Source: CAD feature listing. Evaluate the final solid. Frame: model axes, mm. Coordinates: 2 decimals unless noted, no trailing zeros. Loops run counter-clockwise (first coordinate to the right, second up) from the corner with the lowest first, then second, coordinate; pieces in that order, holes last.
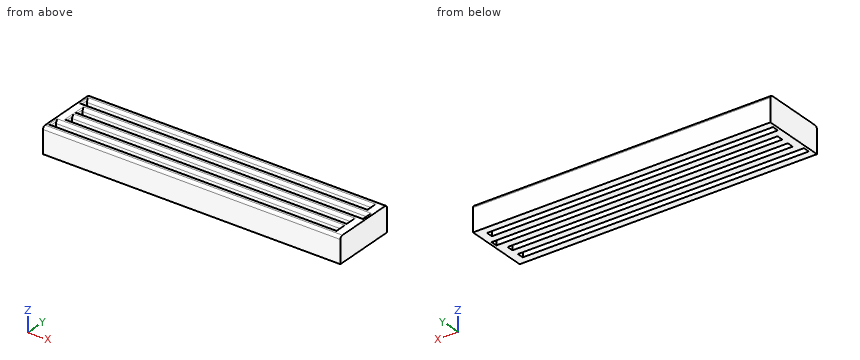
from build123d import *

# Parameters (mm, degrees)
SKETCH003_W   = 53.9
SKETCH003_H   = 11.48
SKETCH003_W_2 = 51.85
SKETCH003_H_2 = 1.194
SKETCH003_W_3 = 50.8
PAD001_DEPTH  = 4.67
FILLET_R      = 0.5
FILLET001_R   = 0.5
FILLET002_R   = 0.5
FILLET003_R   = 0.5
FILLET004_R   = 0.5
FILLET005_R   = 0.5
FILLET006_R   = 0.5
FILLET007_R   = 0.5
FILLET008_R   = 0.5
FILLET009_R   = 0.5
FILLET010_R   = 0.2
FILLET011_R   = 0.2
FILLET012_R   = 0.2
FILLET013_R   = 0.2
FILLET014_R   = 0.2
FILLET015_R   = 0.2
FILLET016_R   = 0.2
FILLET017_R   = 0.19


with BuildPart() as part:
    # Sketch003 → Pad001 (new body)
    with BuildSketch(Plane.XY.offset(0.28)):
        with Locations((27.89, 7.34)):
            Rectangle(SKETCH003_W, SKETCH003_H)
        with Locations((27.365, 11.1422)):
            Rectangle(SKETCH003_W_2, SKETCH003_H_2, mode=Mode.SUBTRACT)
        with Locations((28.415, 8.6074)):
            Rectangle(SKETCH003_W_2, SKETCH003_H_2, mode=Mode.SUBTRACT)
        with Locations((27.89, 6.0726)):
            Rectangle(SKETCH003_W_3, SKETCH003_H_2, mode=Mode.SUBTRACT)
        with Locations((27.365, 3.5378)):
            Rectangle(SKETCH003_W_2, SKETCH003_H_2, mode=Mode.SUBTRACT)
    extrude(amount=PAD001_DEPTH)

    # Fillet
    fillet_edges = [part.edges().sort_by_distance(p)[0] for p in [
        (27.89, 1.6, 4.95),
    ]]
    fillet(fillet_edges, radius=FILLET_R)

    # Fillet001
    fillet001_edges = [part.edges().sort_by_distance(p)[0] for p in [
        (27.365, 2.9408, 4.95),
    ]]
    fillet(fillet001_edges, radius=FILLET001_R)

    # Fillet002
    fillet002_edges = [part.edges().sort_by_distance(p)[0] for p in [
        (27.365, 4.1348, 4.95),
    ]]
    fillet(fillet002_edges, radius=FILLET002_R)

    # Fillet003
    fillet003_edges = [part.edges().sort_by_distance(p)[0] for p in [
        (27.89, 5.4756, 4.95),
    ]]
    fillet(fillet003_edges, radius=FILLET003_R)

    # Fillet004
    fillet004_edges = [part.edges().sort_by_distance(p)[0] for p in [
        (27.89, 6.6696, 4.95),
    ]]
    fillet(fillet004_edges, radius=FILLET004_R)

    # Fillet005
    fillet005_edges = [part.edges().sort_by_distance(p)[0] for p in [
        (28.415, 8.0104, 4.95),
    ]]
    fillet(fillet005_edges, radius=FILLET005_R)

    # Fillet006
    fillet006_edges = [part.edges().sort_by_distance(p)[0] for p in [
        (28.415, 9.2044, 4.95),
    ]]
    fillet(fillet006_edges, radius=FILLET006_R)

    # Fillet007
    fillet007_edges = [part.edges().sort_by_distance(p)[0] for p in [
        (27.365, 10.5452, 4.95),
    ]]
    fillet(fillet007_edges, radius=FILLET007_R)

    # Fillet008
    fillet008_edges = [part.edges().sort_by_distance(p)[0] for p in [
        (27.365, 11.7392, 4.95),
    ]]
    fillet(fillet008_edges, radius=FILLET008_R)

    # Fillet009
    fillet009_edges = [part.edges().sort_by_distance(p)[0] for p in [
        (27.89, 13.08, 4.95),
    ]]
    fillet(fillet009_edges, radius=FILLET009_R)

    # Fillet010
    fillet010_edges = [part.edges().sort_by_distance(p)[0] for p in [
        (53.29, 11.1422, 4.95),
    ]]
    fillet(fillet010_edges, radius=FILLET010_R)

    # Fillet011
    fillet011_edges = [part.edges().sort_by_distance(p)[0] for p in [
        (1.44, 11.1422, 4.95),
    ]]
    fillet(fillet011_edges, radius=FILLET011_R)

    # Fillet012
    fillet012_edges = [part.edges().sort_by_distance(p)[0] for p in [
        (2.49, 8.6074, 4.95),
    ]]
    fillet(fillet012_edges, radius=FILLET012_R)

    # Fillet013
    fillet013_edges = [part.edges().sort_by_distance(p)[0] for p in [
        (54.34, 8.6074, 4.95),
    ]]
    fillet(fillet013_edges, radius=FILLET013_R)

    # Fillet014
    fillet014_edges = [part.edges().sort_by_distance(p)[0] for p in [
        (2.49, 6.0726, 4.95),
    ]]
    fillet(fillet014_edges, radius=FILLET014_R)

    # Fillet015
    fillet015_edges = [part.edges().sort_by_distance(p)[0] for p in [
        (1.44, 3.5378, 4.95),
    ]]
    fillet(fillet015_edges, radius=FILLET015_R)

    # Fillet016
    fillet016_edges = [part.edges().sort_by_distance(p)[0] for p in [
        (53.29, 3.5378, 4.95),
    ]]
    fillet(fillet016_edges, radius=FILLET016_R)

    # Fillet017
    fillet017_edges = [part.edges().sort_by_distance(p)[0] for p in [
        (53.29, 6.0726, 4.95),
    ]]
    fillet(fillet017_edges, radius=FILLET017_R)


solid = part.part
Q1. Line query: line 1 along Y through (x, z) = (42.5, 3.9); line 2 along X through (y, z) = (3.5, 0.5); line 3 along X through (y, z) = (6.5, 0.8). Output: solid intervals per line, ascending.
Q2. Contact query for a flat-ended pin moving along its axis: pin 1 Ø1 at (x, y) = (20, 12) entering from +Z. Output: stop coordinate, or through.
Q3. Section D-D, the plane y = 6. Return the cut outline in (x, z), plus the area to 3 significant figures.
Q4. Section B-B, the plane x = 49. Count the separate pieces of the cut face and the enclosed holes in it, plus the area to 3 significant figures.
Q5. Section A-A, the plane y = 8.75. Return the cut outline in (x, z).
Q6. Section C-C, the plane z = 0.8. Return the cut outline in (x, y).
Derived:
1. line 1: y = 1.6 to 2.94, 4.13 to 5.48, 6.67 to 8.01, 9.2 to 10.55, 11.74 to 13.08
1. line 2: x = 0.94 to 1.44, 53.29 to 54.84
1. line 3: x = 0.94 to 2.49, 53.29 to 54.84
2. pin 1: stops at z = 4.95
3. outline: (0.94, 0.28) - (2.49, 0.28) - (2.49, 4.75) arc R0.2 ccw to (2.29, 4.95) - (0.94, 4.95) - close; (53.29, 0.28) - (54.84, 0.28) - (54.84, 4.95) - (53.48, 4.95) arc R0.19 ccw to (53.29, 4.76) - close
3. area: 14.5 mm2
4. separate pieces: 5
4. enclosed holes: 0
4. area: 30.8 mm2
5. outline: (0.94, 0.28) - (2.49, 0.28) - (2.49, 4.75) arc R0.2 ccw to (2.29, 4.95) - (0.94, 4.95) - close; (54.34, 0.28) - (54.84, 0.28) - (54.84, 4.95) - (54.54, 4.95) arc R0.2 ccw to (54.34, 4.75) - close
6. outline: (0.94, 1.6) - (54.84, 1.6) - (54.84, 13.08) - (0.94, 13.08) - close; hole (1.44, 2.94) - (53.29, 2.94) - (53.29, 4.13) - (1.44, 4.13) - close; hole (1.44, 10.55) - (53.29, 10.55) - (53.29, 11.74) - (1.44, 11.74) - close; hole (2.49, 5.48) - (53.29, 5.48) - (53.29, 6.67) - (2.49, 6.67) - close; hole (2.49, 8.01) - (54.34, 8.01) - (54.34, 9.2) - (2.49, 9.2) - close
